Part model, mm, in its own coordinate system. Give positions to 0.01 mm unless a question says otherwise; leave off trailing zeros. Loops run counter-clockwise (first coordinate to the right, second up) from the corner with the lowest first, then second, coordinate; pieces in that order, holes last. Notation, with made-up numbers: M 9,0.5 L 15,0.5 A12 cw 15,23.5 Z; hole C 44,11 d2. An arc over 180 degrees is marked long. Put each result on its own line as item: value. Start each with the question number.
```python
from build123d import *

# Parameters (mm, degrees)
SKETCH_1_R          = 9.7
EXTRUDE_1_DEPTH     = 4
SKETCH_3_R          = 0.8
CUT_EXTRUDE_1_DEPTH = 10
SKETCH_4_R          = 3
EXTRUDE_2_DEPTH     = 4
SKETCH_5_R          = 1.5
CUT_EXTRUDE_2_DEPTH = 4


with BuildPart() as part:
    # 草图1 → 凸台-拉伸1 (new body)
    with BuildSketch(Plane.XY):
        with BuildLine():
            Line((12.718684308, 6), (286.224480753, 6))
            ThreePointArc((286.224480753, 6), (315.02547605, 0), (286.224480753, -6))
            Line((286.224480753, -6), (12.718684308, -6))
            ThreePointArc((12.718684308, -6), (-14.062891969, 0), (12.718684308, 6))
        make_face()
        Circle(SKETCH_1_R, mode=Mode.SUBTRACT)
        with Locations((300, 0)):
            Circle(SKETCH_1_R, mode=Mode.SUBTRACT)
    extrude(amount=EXTRUDE_1_DEPTH)

    # 草图3 → 切除-拉伸1 (cut)
    with BuildSketch(Plane.XY.offset(4)):
        with Locations((9.7, 0)):
            Circle(SKETCH_3_R)
        with Locations((290.3, 0)):
            Circle(SKETCH_3_R)
    extrude(amount=-CUT_EXTRUDE_1_DEPTH, mode=Mode.SUBTRACT)

    # 草图4 → 凸台-拉伸2 (add)
    with BuildSketch(Plane.XY.offset(4)):
        with Locations((149.47158253, 6)):
            Circle(SKETCH_4_R)
    extrude(amount=-EXTRUDE_2_DEPTH)

    # 草图5 → 切除-拉伸2 (cut)
    with BuildSketch(Plane.XY.offset(4)):
        with Locations((149.47158253, 6)):
            Circle(SKETCH_5_R)
    extrude(amount=-CUT_EXTRUDE_2_DEPTH, mode=Mode.SUBTRACT)


solid = part.part
```
1) Band-saw the part on D-D on x = 213.5. Give the cut face in (y, z), then the cut area to 3 significant figures.
2) Band-saw the part on A-A on x = 300. Give the cut face in (y, z).
3) Wall check: L1, parallel to X at y = 0, z = 1.65; L2, parallel to X at y = -3, z = 0.9; L3, parallel to Y at x = 0, z = 2.2. Give the ranges that are in metal, low to high.
4) Band-saw the part on B-B on z = 2.1. Give the cut face in (x, y), then the cut area to 3 significant figures.
5) Band-saw the part on C-C on x = 0. Give the cut face in (y, z), then the cut area to 3 significant figures.
6) Pin check, flat tips, straight feed: pin 1 Ø1 at (x, z) = (119, 2) entering from +Y; pin 2 Ø1 at (y, z) = (-11, 1) entering from +X; pin 3 Ø2 at (x, z) = (172, 1) entering from -Y. Stop position of each tip, or through.
7) Mould opens along X. For faces 1 (the cylindrical face through (315.014, 0.574, 1.972)), 2 (the flat face through (148, 0, 0)) say: +X half, -X half, draft (parallel to the pull), parting line (faces both ways), or undercut.
Evaluation:
1. outline: M -6,0 L 6,0 L 6,4 L -6,4 Z
1. area: 48.0 mm2
2. outline: M -15.03,0 L -9.7,0 L -9.7,4 L -15.03,4 Z; M 9.7,0 L 15.03,0 L 15.03,4 L 9.7,4 Z
3. L1: -14.06 to -9.7, 10.5 to 289.5, 309.7 to 315.03
3. L2: -13.74 to -9.22, 9.22 to 290.78, 309.22 to 314.72
3. L3: -14.06 to -9.7, 9.7 to 14.06
4. outline: M 12.72,-6 L 286.22,-6 A15.03 ccw long 286.22,6 L 152.47,6 A3 ccw 146.47,6 L 12.72,6 A14.06 ccw long Z; hole M 9.67,-0.8 A0.8 ccw long 9.67,0.8 A9.7 ccw long Z; hole C 149.47,6 d3; hole M 290.33,-0.8 A9.7 ccw long 290.33,0.8 A0.8 ccw long Z
4. area: 4,010 mm2
5. outline: M -14.06,0 L -9.7,0 L -9.7,4 L -14.06,4 Z; M 9.7,0 L 14.06,0 L 14.06,4 L 9.7,4 Z
5. area: 34.9 mm2
6. pin 1: y = 6
6. pin 2: x = 310.75
6. pin 3: y = -6
7. face 1: undercut
7. face 2: draft
